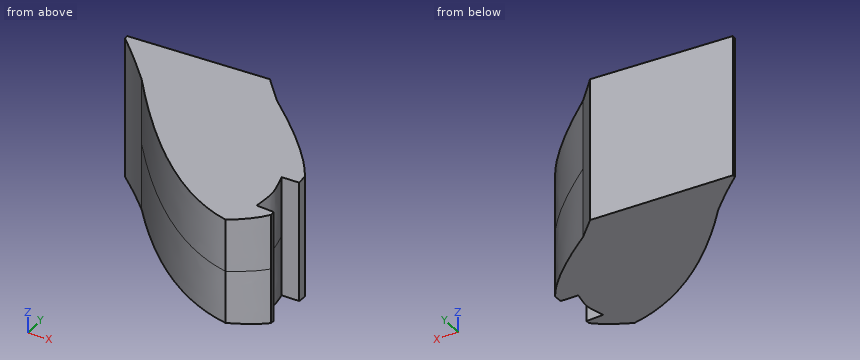
from build123d import *

# Parameters (mm, degrees)
SALIENTE_EXTRUIR1_DEPTH      = 7.5
SALIENTE_EXTRUIR2_DEPTH      = 7.5
SALIENTE_EXTRUIR2_DEPTH_BACK = 7.5
CORTAR_EXTRUIR2_DEPTH        = 28.310606886
CORTAR_EXTRUIR2_DEPTH_BACK   = 28.310606886


with BuildPart() as part:
    # Croquis1 → Saliente-Extruir1 (new, symmetric)
    with BuildSketch(Plane.XY):
        with BuildLine():
            add(Edge.make_bspline(
                [(-18.945192114, 7.540918896), (-10.215008384, -3.697644103), (-2.846604825, -5.059081104)],
                knots=[0.497667241, 0.497667241, 0.497667241, 0.49955428, 0.49955428, 0.49955428], degree=2, weights=[1, 1, 1]))
            add(Edge.make_bspline(
                [(-2.846604825, -5.059081104), (-0.742366882, -3.9352066), (0.355125, -2.723253227)],
                knots=[0.498812075, 0.498812075, 0.498812075, 0.499412845, 0.499412845, 0.499412845], degree=2, weights=[1, 1, 1]))
            Line((0.355125, -2.723253227), (0.355125, -2.284841781))
            Line((0.355125, -2.284841781), (-1.394875, -2.223730435))
            add(Edge.make_bspline(
                [(-1.394875, -2.223730435), (-0.90753067, -0.123730435), (-1.394875, 1.976269565)],
                knots=[0, 0, 0, 1, 1, 1], degree=2, weights=[1, 3.231801219, 1]))
            Line((-1.394875, 1.976269565), (0.355125, 2.284841781))
            Line((0.355125, 2.284841781), (0.355125, 3.001549529))
            add(Edge.make_bspline(
                [(0.355125, 3.001549529), (-1.44872627, 6.058427314), (-6.994875026, 10.477389992)],
                knots=[0.500820705, 0.500820705, 0.500820705, 0.502013312, 0.502013312, 0.502013312], degree=2, weights=[1, 1, 1]))
            Line((-6.994875026, 10.477389992), (-8.981845695, 12.608155172))
            Line((-8.981845695, 12.608155172), (-23.035921146, 11.871612288))
            Line((-23.035921146, 11.871612288), (-23.035921146, 11.54013782))
            ThreePointArc((-23.035921146, 11.54013782), (-20.949684518, 9.582335705), (-18.945192114, 7.540918896))
        make_face()
    extrude(amount=SALIENTE_EXTRUIR1_DEPTH, both=True)

    # Croquis4 → Saliente-Extruir2 (add, two sides: drawn at the far end of the back side and taken through both)
    with BuildSketch(Plane.XY.offset(-SALIENTE_EXTRUIR2_DEPTH_BACK)):
        Polygon((-1.394875, 1.976269565), (0.355125, 2.284841781), (0.355125, 2.037380912), align=None)
    extrude(amount=SALIENTE_EXTRUIR2_DEPTH + SALIENTE_EXTRUIR2_DEPTH_BACK)

    # Croquis6 → Cortar-Extruir2 (cut, two sides: drawn at the far end of the back side and taken through both)
    with BuildSketch(Plane(origin=(0, 0, 0), x_dir=(0, 0, -1), z_dir=(1, 0, 0)).offset(-CORTAR_EXTRUIR2_DEPTH_BACK)):
        Polygon((7.5, 12.608155172), (7.5, -5.059081104), (5.5, -5.059081104), align=None)
        Polygon((-7.5, 12.608155172), (-7.5, -5.059081104), (-5.5, -5.059081104), align=None)
    extrude(amount=CORTAR_EXTRUIR2_DEPTH + CORTAR_EXTRUIR2_DEPTH_BACK, mode=Mode.SUBTRACT)


solid = part.part
Design review of the part built by this model. Coordinates are the model's own, in mm. Give positions to 0.01 mm unless a question says otherwise; leave off trailing zeros. Loops run counter-clockwise (first coordinate to the right, second up) from the corner with the lowest first, then second, coordinate; pieces in that order, holes last. Notation, with made-up numbers: (51, 40.5) -> (65, 40.5) arc R28 cw to (65, 77.5) -> close; hole circle Ø1 at (9, -2.75). An arc over 180 degrees is marked (long way). One line per question, with ' | ' between items. Start each with the question number.
(1) For line 1 (X direction, y = 11.5, z = -4); line 2 (X direction, y = 9.25, z = 6.25); line 3 (Y direction, x = -18.5, z = -0.25), list the stretches that pass through material, from the lowest coordinate up.
(2) We need section A-A (x = -21). State the section outline as (y, z) points.
(3) Insertion check: P1, Ø5, axis at x = -20, y = 8.5, coming from the +Z side; P2, Ø6, axis at y = 1, z = 5.5, coming from the -X side; P3, Ø1, axis at y = -1.5, z = 3, coming from the -X side. Each pin has a flat end and moves straight along its axis. Give the tip position at first contact, or say it passes through.
The answers:
1) line 1: x = -22.99 to -7.95 | line 2: x = -20.61 to -5.5 | line 3: y = 6.97 to 12.11
2) outline: (9.63, -7.16) -> (11.98, -7.43) -> (11.98, 7.43) -> (9.63, 7.16) -> close
3) P1: stops at z = 7.32 | P2: stops at x = -16.01 | P3: stops at x = -10.84
